Source: CAD feature listing. Evaluate the final solid. Frame: model axes, mm. Coordinates: 2 decimals unless noted, no trailing zeros. Order: outer loops, then holes, each group sorted by start corner. A loop starts at its lowest first (then second) coordinate and runs counter-clockwise, first axis right, second up. Notation, with made-up numbers: (10, 25.5) - (41, 25.5) arc R21 ccw to (41, 32.5) - close; hole circle Ø7 at (44, 77). An arc over 180 degrees is marked (long way). One line per question, with ' | ' between items.
from build123d import *

# Parameters (mm, degrees)
SKETCH1_R           = 1.05
BOSS_EXTRUDE3_DEPTH = 2


with BuildPart() as part:
    # Sketch1 → Boss-Extrude3 (new body)
    with BuildSketch(Plane.XY):
        with BuildLine():
            Line((12.837896157, 8.299592267), (12.178844101, 8.362202212))
            ThreePointArc((12.178844101, 8.362202212), (8.678844101, 4.862202212), (12.178844101, 1.362202212))
            Line((12.178844101, 1.362202212), (12.837896157, 1.424812158))
            Line((12.837896157, 1.424812158), (22.178844101, 2.312202212))
            ThreePointArc((22.178844101, 2.312202212), (24.728844101, 4.862202212), (22.178844101, 7.412202212))
            Line((22.178844101, 7.412202212), (12.837896157, 8.299592267))
        make_face()
        with BuildLine():
            Line((11.619157127, 2.552399344), (11.653043843, 3.328532726))
            ThreePointArc((11.653043843, 3.328532726), (11.575639379, 3.40593719), (11.466172936, 3.40593719))
            Line((11.466172936, 3.40593719), (10.941325284, 2.833166486))
            Line((10.941325284, 2.833166486), (10.767566215, 2.643541736))
            ThreePointArc((10.767566215, 2.643541736), (10.717983865, 2.675870364), (10.669141763, 2.709306852))
            Line((10.669141763, 2.709306852), (10.777837472, 2.94240555))
            Line((10.777837472, 2.94240555), (11.106158101, 3.646491412))
            ThreePointArc((11.106158101, 3.646491412), (11.064267107, 3.747625218), (10.963133301, 3.789516212))
            Line((10.963133301, 3.789516212), (10.259047439, 3.461195582))
            Line((10.259047439, 3.461195582), (10.025948741, 3.352499874))
            ThreePointArc((10.025948741, 3.352499874), (9.992512253, 3.401341976), (9.960183625, 3.450924326))
            Line((9.960183625, 3.450924326), (10.149808375, 3.624683395))
            Line((10.149808375, 3.624683395), (10.722579079, 4.149531047))
            ThreePointArc((10.722579079, 4.149531047), (10.722579079, 4.258997489), (10.645174615, 4.336401953))
            Line((10.645174615, 4.336401953), (9.869041233, 4.302515238))
            Line((9.869041233, 4.302515238), (9.61209007, 4.291296508))
            ThreePointArc((9.61209007, 4.291296508), (9.599889846, 4.349216316), (9.588996432, 4.407396064))
            Line((9.588996432, 4.407396064), (9.830681575, 4.495362262))
            Line((9.830681575, 4.495362262), (10.560703205, 4.761068406))
            ThreePointArc((10.560703205, 4.761068406), (10.602594199, 4.862202212), (10.560703205, 4.963336018))
            Line((10.560703205, 4.963336018), (9.830681575, 5.229042162))
            Line((9.830681575, 5.229042162), (9.588996432, 5.31700836))
            ThreePointArc((9.588996432, 5.31700836), (9.599889846, 5.375188109), (9.61209007, 5.433107916))
            Line((9.61209007, 5.433107916), (9.869041233, 5.421889186))
            Line((9.869041233, 5.421889186), (10.645174615, 5.388002471))
            ThreePointArc((10.645174615, 5.388002471), (10.722579079, 5.465406935), (10.722579079, 5.574873378))
            Line((10.722579079, 5.574873378), (10.149808375, 6.099721029))
            Line((10.149808375, 6.099721029), (9.960183625, 6.273480099))
            ThreePointArc((9.960183625, 6.273480099), (9.992512253, 6.323062449), (10.025948741, 6.37190455))
            Line((10.025948741, 6.37190455), (10.259047439, 6.263208842))
            Line((10.259047439, 6.263208842), (10.963133301, 5.934888213))
            ThreePointArc((10.963133301, 5.934888213), (11.064267107, 5.976779207), (11.106158101, 6.077913013))
            Line((11.106158101, 6.077913013), (10.777837472, 6.781998874))
            Line((10.777837472, 6.781998874), (10.669141763, 7.015097573))
            ThreePointArc((10.669141763, 7.015097573), (10.717983865, 7.048534061), (10.767566215, 7.080862689))
            Line((10.767566215, 7.080862689), (10.941325284, 6.891237939))
            Line((10.941325284, 6.891237939), (11.466172936, 6.318467235))
            ThreePointArc((11.466172936, 6.318467235), (11.575639379, 6.318467235), (11.653043843, 6.395871699))
            Line((11.653043843, 6.395871699), (11.619157127, 7.172005081))
            Line((11.619157127, 7.172005081), (11.607938397, 7.428956244))
            ThreePointArc((11.607938397, 7.428956244), (11.665858205, 7.441156468), (11.724037954, 7.452049882))
            Line((11.724037954, 7.452049882), (11.812004151, 7.210364739))
            Line((11.812004151, 7.210364739), (12.077710295, 6.480343109))
            ThreePointArc((12.077710295, 6.480343109), (12.178844101, 6.438452114), (12.279977907, 6.480343109))
            Line((12.279977907, 6.480343109), (12.545684051, 7.210364739))
            Line((12.545684051, 7.210364739), (12.633650249, 7.452049882))
            ThreePointArc((12.633650249, 7.452049882), (12.691829998, 7.441156468), (12.749749805, 7.428956244))
            Line((12.749749805, 7.428956244), (12.738531075, 7.172005081))
            Line((12.738531075, 7.172005081), (12.70464436, 6.395871699))
            ThreePointArc((12.70464436, 6.395871699), (12.782048824, 6.318467235), (12.891515267, 6.318467235))
            Line((12.891515267, 6.318467235), (13.416362918, 6.891237939))
            Line((13.416362918, 6.891237939), (13.590121988, 7.080862689))
            ThreePointArc((13.590121988, 7.080862689), (13.639704338, 7.048534061), (13.688546439, 7.015097573))
            Line((13.688546439, 7.015097573), (13.579850731, 6.781998874))
            Line((13.579850731, 6.781998874), (13.251530102, 6.077913013))
            ThreePointArc((13.251530102, 6.077913013), (13.293421096, 5.976779207), (13.394554902, 5.934888213))
            Line((13.394554902, 5.934888213), (14.098640763, 6.263208842))
            Line((14.098640763, 6.263208842), (14.331739462, 6.37190455))
            ThreePointArc((14.331739462, 6.37190455), (14.36517595, 6.323062449), (14.397504578, 6.273480099))
            Line((14.397504578, 6.273480099), (14.207879828, 6.099721029))
            Line((14.207879828, 6.099721029), (13.635109124, 5.574873378))
            ThreePointArc((13.635109124, 5.574873378), (13.635109124, 5.465406935), (13.712513588, 5.388002471))
            Line((13.712513588, 5.388002471), (14.48864697, 5.421889186))
            Line((14.48864697, 5.421889186), (14.745598133, 5.433107916))
            ThreePointArc((14.745598133, 5.433107916), (14.757798357, 5.375188109), (14.768691771, 5.31700836))
            Line((14.768691771, 5.31700836), (14.527006628, 5.229042162))
            Line((14.527006628, 5.229042162), (13.796984998, 4.963336018))
            ThreePointArc((13.796984998, 4.963336018), (13.755094004, 4.862202212), (13.796984998, 4.761068406))
            Line((13.796984998, 4.761068406), (14.527006628, 4.495362262))
            Line((14.527006628, 4.495362262), (14.768691771, 4.407396064))
            ThreePointArc((14.768691771, 4.407396064), (14.757798357, 4.349216316), (14.745598133, 4.291296508))
            Line((14.745598133, 4.291296508), (14.48864697, 4.302515238))
            Line((14.48864697, 4.302515238), (13.712513588, 4.336401953))
            ThreePointArc((13.712513588, 4.336401953), (13.635109124, 4.258997489), (13.635109124, 4.149531047))
            Line((13.635109124, 4.149531047), (14.207879828, 3.624683395))
            Line((14.207879828, 3.624683395), (14.397504578, 3.450924326))
            ThreePointArc((14.397504578, 3.450924326), (14.36517595, 3.401341976), (14.331739462, 3.352499874))
            Line((14.331739462, 3.352499874), (14.098640763, 3.461195582))
            Line((14.098640763, 3.461195582), (13.394554902, 3.789516212))
            ThreePointArc((13.394554902, 3.789516212), (13.293421096, 3.747625218), (13.251530102, 3.646491412))
            Line((13.251530102, 3.646491412), (13.579850731, 2.94240555))
            Line((13.579850731, 2.94240555), (13.688546439, 2.709306852))
            ThreePointArc((13.688546439, 2.709306852), (13.639704338, 2.675870364), (13.590121988, 2.643541736))
            Line((13.590121988, 2.643541736), (13.416362918, 2.833166486))
            Line((13.416362918, 2.833166486), (12.891515267, 3.40593719))
            ThreePointArc((12.891515267, 3.40593719), (12.782048824, 3.40593719), (12.70464436, 3.328532726))
            Line((12.70464436, 3.328532726), (12.738531075, 2.552399344))
            Line((12.738531075, 2.552399344), (12.749749805, 2.295448181))
            ThreePointArc((12.749749805, 2.295448181), (12.691829998, 2.283247957), (12.633650249, 2.272354543))
            Line((12.633650249, 2.272354543), (12.545684051, 2.514039686))
            Line((12.545684051, 2.514039686), (12.279977907, 3.244061316))
            ThreePointArc((12.279977907, 3.244061316), (12.178844101, 3.28595231), (12.077710295, 3.244061316))
            Line((12.077710295, 3.244061316), (11.812004151, 2.514039686))
            Line((11.812004151, 2.514039686), (11.724037954, 2.272354543))
            ThreePointArc((11.724037954, 2.272354543), (11.665858205, 2.283247957), (11.607938397, 2.295448181))
            Line((11.607938397, 2.295448181), (11.619157127, 2.552399344))
        make_face(mode=Mode.SUBTRACT)
        with Locations((22.178844101, 4.862202212)):
            Circle(SKETCH1_R, mode=Mode.SUBTRACT)
    extrude(amount=BOSS_EXTRUDE3_DEPTH)


solid = part.part
(1) Cut plane A-A (z = 0.2). State how many separate pieces and enclosed holes the cut face has, and give its area (3 significant figures).
Taken from the geometry:
separate pieces: 1 | enclosed holes: 2 | area: 73.9 mm²
(2) Pull-direction query (Y, two-part tool) for faces 1 (the cylindrical face through (21.13, 4.91, 0.99)), 2 (the cylindrical face through (24.73, 4.81, 0.99)), 3 (the flat face through (17, 5, 0)); classes: pulls with the +Y half, pulls with the -Y half, needs draft (parallel to the pull), parting line crosses it, or undercut.
Taken from the geometry:
face 1: undercut | face 2: parting line crosses it | face 3: needs draft
(3) Cut plane C-C (x = 23.5). Return the cut outline in (y, z).
Taken from the geometry:
outline: (2.68, 0) - (7.04, 0) - (7.04, 2) - (2.68, 2) - close
(4) Pin query (flat end, axial travel): P1, Ø1.3, axis at x = 22.18, y = 4.86, coming from the -Z side. Return the tip coordinate at first contact, or that it passes through.
Taken from the geometry:
P1: passes through
(5) Cut plane B-B (x = 16.75). Return the cut outline in (y, z).
Taken from the geometry:
outline: (1.8, 0) - (7.93, 0) - (7.93, 2) - (1.8, 2) - close
(6) Material intervals for L1, parallel to Y at x = 11, z = 1.8; L2, parallel to Y at x = 10.5, z = 0.1; L3, parallel to X at y = 4, z = 0.6, sorted ascending. Write a range as from..to.
Taken from the geometry:
L1: y = 1.57..2.9, 3.42..3.78, 5.94..6.31, 6.83..8.16 | L2: y = 1.79..3.57, 3.95..4.33, 4.74..4.99, 5.39..5.78, 6.15..7.93 | L3: x = 8.79..10.56, 13.8..21.58, 22.78..24.58
